For this review, use the dimensioned drawing (mm, ordinates from the lowest corner) and the shaded views. A direction names the side the tool comes from. Coordinates: 2 decimals unless noted, no trailing zeros. Order: outer loops, then holes, each group sorted by start corner. A loop starts at its lowest first (then second) coordinate and runs counter-clockwise, first axis right, second up. Notation, with made-up numbers: M -28.75,-36.75 L 11.25,-36.75 A32 cw 11.25,2.25 Z; hole C -8,28.25 d3. An arc over 180 degrees is marked long. Use CSV: the item, a comma, the result in double quotes.
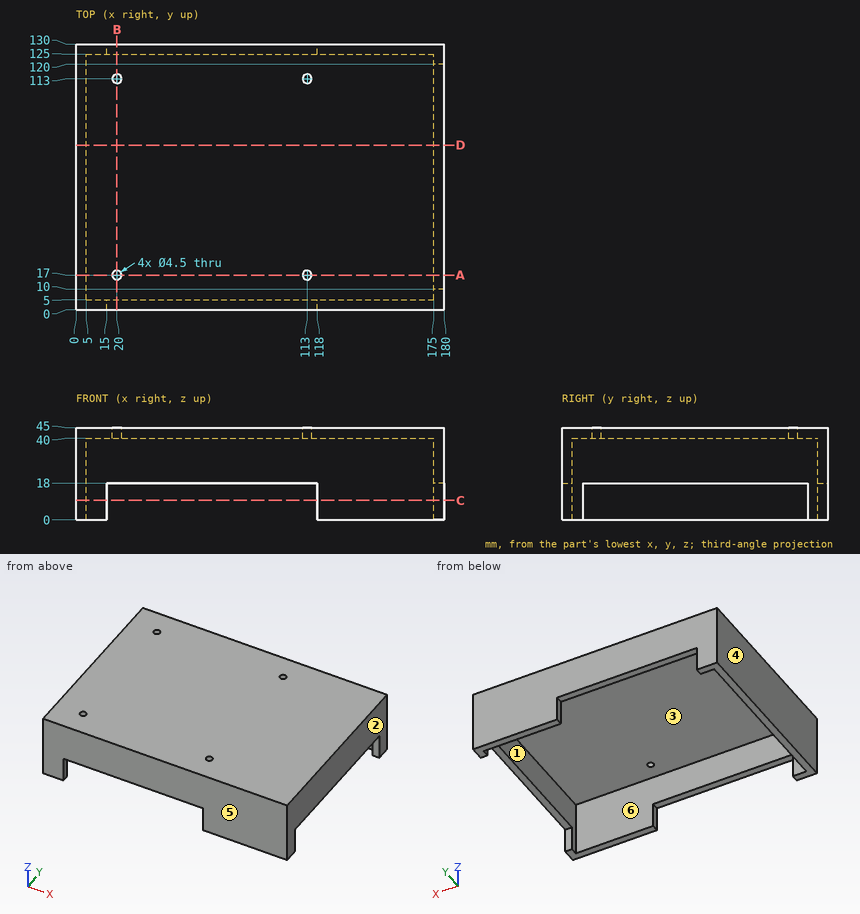
Item 1: Add section C-C on z = 9.5. State the section outline as (x, y) points, and give its area (3 significant figures).
Solutions:
outline,"M 0,0 L 15,0 L 15,5 L 5,5 L 5,125 L 15,125 L 15,130 L 0,130 Z; M 118,0 L 180,0 L 180,10 L 175,10 L 175,5 L 118,5 Z; M 118,125 L 175,125 L 175,120 L 180,120 L 180,130 L 118,130 Z"
area,"1,420 mm^2"
Item 2: Clearance check with flat-ended pins moving along their axes: pin 1 Ø2.5 at (x, y) = (66, 2) entering from -Z; pin 2 Ø4 at (y, z) = (13, 9) entering from +X. State where each tip first meets the part, or that it passes through.
Solutions:
pin 1,"z = 18"
pin 2,"x = 5"
Item 3: For the marked faces 1 and 2, list the 3-axis set-ups (+Z, -Z, +X, -X, +Y, -Y) from which the entire face can be reached by the end or side of a thin tool; tool diameter is ignored.
Solutions:
face 1,"-Z"
face 2,"+Z, -Z, +X, +Y, -Y"
Item 4: Add section D-D on y = 80.5. State the section outline as (x, z) points, and give its area (3 significant figures).
Solutions:
outline,"M 0,0 L 5,0 L 5,40 L 175,40 L 175,18 L 180,18 L 180,45 L 0,45 Z"
area,"1,210 mm^2"
Item 5: Add section B-B on x = 20. State the section outline as (y, z) points, and give its area (3 significant figures).
Solutions:
outline,"M 0,18 L 5,18 L 5,40 L 14.75,40 L 14.75,45 L 0,45 Z; M 19.25,40 L 110.75,40 L 110.75,45 L 19.25,45 Z; M 115.25,40 L 125,40 L 125,18 L 130,18 L 130,45 L 115.25,45 Z"
area,"825 mm^2"
Item 6: To check wall thickness, follow line 1 along Y through (x, z) = (113, 43.9); line 2 along Y through (x, z) = (8, 21.5); line 3 along X through (y, z) = (109, 38). State the ranges of each line that lie inside material, in increasing order. Write a range as [from, to].
Solutions:
line 1,"[0, 14.75], [19.25, 110.75], [115.25, 130]"
line 2,"[0, 5], [125, 130]"
line 3,"[0, 5], [175, 180]"
Item 7: Draft analysis for pull direction Y (two halves, no side actions). For the marked faces 3, 4, 5 and 6, state which applies: released by +Y, released by -Y, zero draft, split by the parting line, or undercut.
Solutions:
face 3,"undercut"
face 4,"zero draft"
face 5,"released by -Y"
face 6,"undercut"
Item 8: Add section A-A on y = 17. State the section outline as (x, z) points.
Solutions:
outline,"M 0,0 L 5,0 L 5,40 L 17.75,40 L 17.75,45 L 0,45 Z; M 22.25,40 L 110.75,40 L 110.75,45 L 22.25,45 Z; M 115.25,40 L 175,40 L 175,18 L 180,18 L 180,45 L 115.25,45 Z"
